Could you check a few things on this model? Use its own coordinates, in mm. Round coordinates to 2 decimals unless told otherwise and drop trailing zeros. Write each loop counter-clockwise with the first axis right and the second up, starting at its lowest first coordinate (ties: lowest second). Pieces come first, ordered by that corner, then holes. Notation, with made-up numbers: (-15.75, 77) -> (1.25, 77) arc R23 cw to (1.25, 115) -> close; hole circle Ø5 at (87.25, 74). An arc over 180 degrees is marked (long way). One line per question, with ' | ' between items. Start each with the question number.
1. Imagine slicing it at A-A, the plane x = 3. List the corners of the cut face in (y, z) for me.
2. Imagine slicing it at B-B, the plane x = 70. List the corners of the cut face in (y, z) for me.
3. For pin 1 Ø1.6 at (x, y) = (3, 19.5) entering from +Z, with a flat end and sliding along its axis, tell me the tip position at first contact or that it passes through.
4. If I drill on line 1 along Y through (x, z) = (63, 0.2); line 2 along Y through (x, z) = (35, 0.1); line 3 along Y through (x, z) = (50.5, 0.25), over which ranges is the centre line in solid material (lowest first)? Write a range as [from, to].
from build123d import *

# Parameters (mm, degrees)
BOARD_DEPTH                        = 0.41148
F_1_0_228_DIAMETER_HOLE1_OUTLINE_R = 0.4572
F_1_0_228_DIAMETER_HOLE1_DEPTH     = 0.41148
F_1_0_228_DIAMETER_HOLE2_OUTLINE_R = 0.4318
F_1_0_228_DIAMETER_HOLE2_DEPTH     = 0.41148
SKETCH6_R                          = 0.999998
CUT_EXTRUDE1_DEPTH                 = 77.389914621
SKETCH7_R                          = 0.999998
CUT_EXTRUDE2_DEPTH                 = 77.389914621
SKETCH8_R                          = 0.999998
CUT_EXTRUDE3_DEPTH                 = 77.389914621
SKETCH9_R                          = 0.999998
CUT_EXTRUDE4_DEPTH                 = 77.389914621
SKETCH10_R                         = 0.999998
CUT_EXTRUDE5_DEPTH                 = 77.389914621


# Read off the part's stored shape, not the designer's step: #1 (0.228) Diameter Hole1, #1 (0.228) Diameter Hole2
with BuildPart() as part:
    # Sketch1 → Board (new body)
    with BuildSketch(Plane.XY):
        with BuildLine():
            Line((0.999998, 22.49999818), (71.99999824, 22.49999564))
            ThreePointArc((71.99999824, 22.49999564), (72.707104877, 22.207103533), (72.99999878, 21.49999764))
            Line((72.99999878, 21.49999764), (72.99999624, -1.2499975))
            ThreePointArc((72.99999624, -1.2499975), (72.707104133, -1.957104137), (71.99999824, -2.24999804))
            Line((71.99999824, -2.24999804), (54.74999972, -2.25000058))
            ThreePointArc((54.74999972, -2.25000058), (54.042893083, -2.542892687), (53.74999918, -3.24999858))
            Line((53.74999918, -3.24999858), (53.74999664, -15.49999948))
            ThreePointArc((53.74999664, -15.49999948), (53.457104007, -16.207104847), (52.74999864, -16.49999748))
            Line((52.74999864, -16.49999748), (23.74999822, -16.49999748))
            ThreePointArc((23.74999822, -16.49999748), (23.042891583, -16.207105373), (22.74999768, -15.49999948))
            Line((22.74999768, -15.49999948), (22.74999768, -0.999998))
            ThreePointArc((22.74999768, -0.999998), (22.457105047, -0.292892633), (21.74999968, 0))
            Line((21.74999968, 0), (0.999998, 0))
            ThreePointArc((0.999998, 0), (0.292892633, 0.292892633), (0, 0.999998))
            Line((0, 0.999998), (-2.54e-06, 21.49999764))
            ThreePointArc((-2.54e-06, 21.49999764), (0.292890837, 22.207104803), (0.999998, 22.49999818))
        make_face()
    extrude(amount=BOARD_DEPTH)

    # #1 (0.228) Diameter Hole1 outline → #1 (0.228) Diameter Hole1 (cut)
    with BuildSketch(Plane.XY):
        with Locations((37.62799942, 16.24500434)):
            Circle(F_1_0_228_DIAMETER_HOLE1_OUTLINE_R)
        with Locations((40.16799942, 16.24500434)):
            Circle(F_1_0_228_DIAMETER_HOLE1_OUTLINE_R)
        with Locations((42.70799942, 16.24500434)):
            Circle(F_1_0_228_DIAMETER_HOLE1_OUTLINE_R)
        with Locations((45.24799942, 16.24500434)):
            Circle(F_1_0_228_DIAMETER_HOLE1_OUTLINE_R)
        with Locations((47.78799942, 16.24500434)):
            Circle(F_1_0_228_DIAMETER_HOLE1_OUTLINE_R)
        with Locations((50.32799942, 16.24500434)):
            Circle(F_1_0_228_DIAMETER_HOLE1_OUTLINE_R)
        with Locations((52.86799942, 16.24500434)):
            Circle(F_1_0_228_DIAMETER_HOLE1_OUTLINE_R)
        with Locations((55.40799942, 16.24500434)):
            Circle(F_1_0_228_DIAMETER_HOLE1_OUTLINE_R)
        with Locations((57.94799942, 16.24500434)):
            Circle(F_1_0_228_DIAMETER_HOLE1_OUTLINE_R)
        with Locations((60.48799942, 16.24500434)):
            Circle(F_1_0_228_DIAMETER_HOLE1_OUTLINE_R)
        with Locations((63.02799942, 16.24500434)):
            Circle(F_1_0_228_DIAMETER_HOLE1_OUTLINE_R)
        with Locations((65.56799942, 16.24500434)):
            Circle(F_1_0_228_DIAMETER_HOLE1_OUTLINE_R)
        with Locations((65.56799942, 3.54500434)):
            Circle(F_1_0_228_DIAMETER_HOLE1_OUTLINE_R)
        with Locations((63.02799942, 3.54500434)):
            Circle(F_1_0_228_DIAMETER_HOLE1_OUTLINE_R)
        with Locations((60.48799942, 3.54500434)):
            Circle(F_1_0_228_DIAMETER_HOLE1_OUTLINE_R)
        with Locations((57.94799942, 3.54500434)):
            Circle(F_1_0_228_DIAMETER_HOLE1_OUTLINE_R)
        with Locations((55.40799942, 3.54500434)):
            Circle(F_1_0_228_DIAMETER_HOLE1_OUTLINE_R)
        with Locations((52.86799942, 3.54500434)):
            Circle(F_1_0_228_DIAMETER_HOLE1_OUTLINE_R)
        with Locations((50.32799942, 3.54500434)):
            Circle(F_1_0_228_DIAMETER_HOLE1_OUTLINE_R)
        with Locations((47.78799942, 3.54500434)):
            Circle(F_1_0_228_DIAMETER_HOLE1_OUTLINE_R)
        with Locations((45.24799942, 3.54500434)):
            Circle(F_1_0_228_DIAMETER_HOLE1_OUTLINE_R)
        with Locations((42.70799942, 3.54500434)):
            Circle(F_1_0_228_DIAMETER_HOLE1_OUTLINE_R)
        with Locations((40.16799942, 3.54500434)):
            Circle(F_1_0_228_DIAMETER_HOLE1_OUTLINE_R)
        with Locations((37.62799942, 3.54500434)):
            Circle(F_1_0_228_DIAMETER_HOLE1_OUTLINE_R)
        with Locations((7.42800902, 16.24500434)):
            Circle(F_1_0_228_DIAMETER_HOLE1_OUTLINE_R)
        with Locations((9.96800902, 16.24500434)):
            Circle(F_1_0_228_DIAMETER_HOLE1_OUTLINE_R)
        with Locations((12.50800902, 16.24500434)):
            Circle(F_1_0_228_DIAMETER_HOLE1_OUTLINE_R)
        with Locations((15.04800902, 16.24500434)):
            Circle(F_1_0_228_DIAMETER_HOLE1_OUTLINE_R)
        with Locations((17.58800902, 16.24500434)):
            Circle(F_1_0_228_DIAMETER_HOLE1_OUTLINE_R)
        with Locations((20.12800902, 16.24500434)):
            Circle(F_1_0_228_DIAMETER_HOLE1_OUTLINE_R)
        with Locations((22.66800902, 16.24500434)):
            Circle(F_1_0_228_DIAMETER_HOLE1_OUTLINE_R)
        with Locations((25.20800902, 16.24500434)):
            Circle(F_1_0_228_DIAMETER_HOLE1_OUTLINE_R)
        with Locations((27.74800902, 16.24500434)):
            Circle(F_1_0_228_DIAMETER_HOLE1_OUTLINE_R)
        with Locations((30.28800902, 16.24500434)):
            Circle(F_1_0_228_DIAMETER_HOLE1_OUTLINE_R)
        with Locations((32.82800902, 16.24500434)):
            Circle(F_1_0_228_DIAMETER_HOLE1_OUTLINE_R)
        with Locations((35.36800902, 16.24500434)):
            Circle(F_1_0_228_DIAMETER_HOLE1_OUTLINE_R)
        with Locations((35.36800902, 3.54500434)):
            Circle(F_1_0_228_DIAMETER_HOLE1_OUTLINE_R)
        with Locations((32.82800902, 3.54500434)):
            Circle(F_1_0_228_DIAMETER_HOLE1_OUTLINE_R)
        with Locations((30.28800902, 3.54500434)):
            Circle(F_1_0_228_DIAMETER_HOLE1_OUTLINE_R)
        with Locations((27.74800902, 3.54500434)):
            Circle(F_1_0_228_DIAMETER_HOLE1_OUTLINE_R)
        with Locations((25.20800902, 3.54500434)):
            Circle(F_1_0_228_DIAMETER_HOLE1_OUTLINE_R)
        with Locations((22.66800902, 3.54500434)):
            Circle(F_1_0_228_DIAMETER_HOLE1_OUTLINE_R)
        with Locations((20.12800902, 3.54500434)):
            Circle(F_1_0_228_DIAMETER_HOLE1_OUTLINE_R)
        with Locations((17.58800902, 3.54500434)):
            Circle(F_1_0_228_DIAMETER_HOLE1_OUTLINE_R)
        with Locations((15.04800902, 3.54500434)):
            Circle(F_1_0_228_DIAMETER_HOLE1_OUTLINE_R)
        with Locations((12.50800902, 3.54500434)):
            Circle(F_1_0_228_DIAMETER_HOLE1_OUTLINE_R)
        with Locations((9.96800902, 3.54500434)):
            Circle(F_1_0_228_DIAMETER_HOLE1_OUTLINE_R)
        with Locations((7.42800902, 3.54500434)):
            Circle(F_1_0_228_DIAMETER_HOLE1_OUTLINE_R)
    extrude(amount=F_1_0_228_DIAMETER_HOLE1_DEPTH, mode=Mode.SUBTRACT)

    # #1 (0.228) Diameter Hole2 outline → #1 (0.228) Diameter Hole2 (cut)
    with BuildSketch(Plane.XY):
        with Locations((47.15000222, -6.81499526)):
            Circle(F_1_0_228_DIAMETER_HOLE2_OUTLINE_R)
        with Locations((47.15000222, -9.35499526)):
            Circle(F_1_0_228_DIAMETER_HOLE2_OUTLINE_R)
        with Locations((44.61000222, -6.81499526)):
            Circle(F_1_0_228_DIAMETER_HOLE2_OUTLINE_R)
        with Locations((44.61000222, -9.35499526)):
            Circle(F_1_0_228_DIAMETER_HOLE2_OUTLINE_R)
        with Locations((42.07000222, -6.81499526)):
            Circle(F_1_0_228_DIAMETER_HOLE2_OUTLINE_R)
        with Locations((42.07000222, -9.35499526)):
            Circle(F_1_0_228_DIAMETER_HOLE2_OUTLINE_R)
        with Locations((39.53000222, -6.81499526)):
            Circle(F_1_0_228_DIAMETER_HOLE2_OUTLINE_R)
        with Locations((39.53000222, -9.35499526)):
            Circle(F_1_0_228_DIAMETER_HOLE2_OUTLINE_R)
        with Locations((36.99000222, -6.81499526)):
            Circle(F_1_0_228_DIAMETER_HOLE2_OUTLINE_R)
        with Locations((36.99000222, -9.35499526)):
            Circle(F_1_0_228_DIAMETER_HOLE2_OUTLINE_R)
        with Locations((34.45000222, -6.81499526)):
            Circle(F_1_0_228_DIAMETER_HOLE2_OUTLINE_R)
        with Locations((34.45000222, -9.35499526)):
            Circle(F_1_0_228_DIAMETER_HOLE2_OUTLINE_R)
        with Locations((31.91000222, -6.81499526)):
            Circle(F_1_0_228_DIAMETER_HOLE2_OUTLINE_R)
        with Locations((31.91000222, -9.35499526)):
            Circle(F_1_0_228_DIAMETER_HOLE2_OUTLINE_R)
        with Locations((29.37000222, -6.81499526)):
            Circle(F_1_0_228_DIAMETER_HOLE2_OUTLINE_R)
        with Locations((29.37000222, -9.35499526)):
            Circle(F_1_0_228_DIAMETER_HOLE2_OUTLINE_R)
    extrude(amount=F_1_0_228_DIAMETER_HOLE2_DEPTH, mode=Mode.SUBTRACT)

    # Sketch6 → Cut-Extrude1 (cut, through all)
    with BuildSketch(Plane.XY.offset(0.41148)):
        with Locations((50.24999856, -14.49999894)):
            Circle(SKETCH6_R)
    extrude(amount=-CUT_EXTRUDE1_DEPTH, mode=Mode.SUBTRACT)

    # Sketch7 → Cut-Extrude2 (cut, through all)
    with BuildSketch(Plane.XY.offset(0.41148)):
        with Locations((2.99999908, 19.4999991)):
            Circle(SKETCH7_R)
    extrude(amount=-CUT_EXTRUDE2_DEPTH, mode=Mode.SUBTRACT)

    # Sketch8 → Cut-Extrude3 (cut, through all)
    with BuildSketch(Plane.XY.offset(0.41148)):
        with Locations((48.99999852, 20.49999964)):
            Circle(SKETCH8_R)
    extrude(amount=-CUT_EXTRUDE3_DEPTH, mode=Mode.SUBTRACT)

    # Sketch9 → Cut-Extrude4 (cut, through all)
    with BuildSketch(Plane.XY.offset(0.41148)):
        with Locations((69.9999997, 0.999998)):
            Circle(SKETCH9_R)
    extrude(amount=-CUT_EXTRUDE4_DEPTH, mode=Mode.SUBTRACT)

    # Sketch10 → Cut-Extrude5 (cut, through all)
    with BuildSketch(Plane.XY.offset(0.41148)):
        with Locations((26.4999978, -0.999998)):
            Circle(SKETCH10_R)
    extrude(amount=-CUT_EXTRUDE5_DEPTH, mode=Mode.SUBTRACT)


solid = part.part
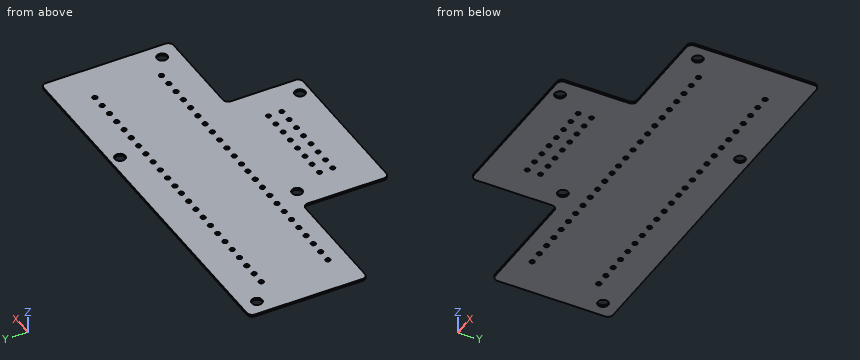
Geometry results:
1) outline: (0, 0) -> (18.5, 0) -> (18.5, 0.41) -> (0, 0.41) -> close; (20.5, 0) -> (22.5, 0) -> (22.5, 0.41) -> (20.5, 0.41) -> close
2) outline: (-2.25, 0) -> (0, 0) -> (0, 0.41) -> (-2.25, 0.41) -> close; (2, 0) -> (22.5, 0) -> (22.5, 0.41) -> (2, 0.41) -> close
3) pin 1: passes through
4) line 1: y = [-2.25, 3.09], [4, 15.79], [16.7, 22.5] | line 2: y = [-16.5, 3.27], [3.82, 15.97], [16.52, 22.5] | line 3: y = [-16.5, -15.47], [-13.53, 3.12], [3.97, 15.82], [16.67, 22.5]
